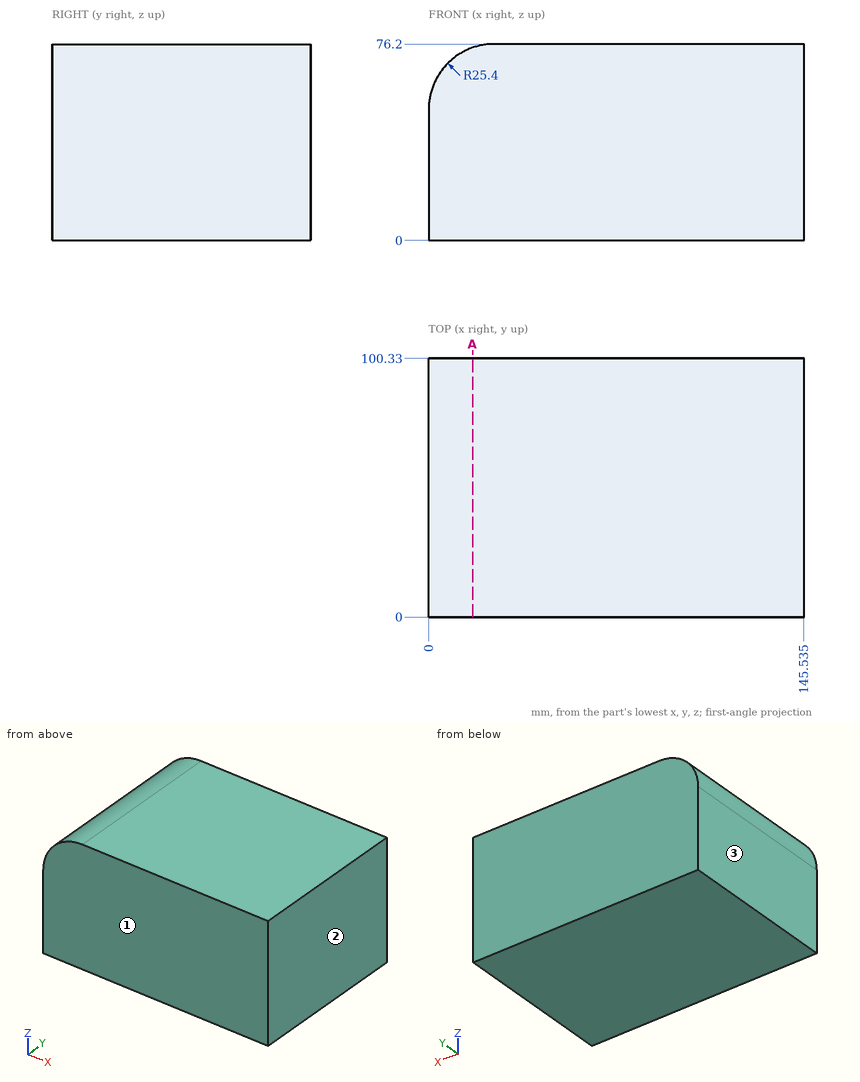
Part print with two shaded views. Sizes in mm from the minimum x, y, z corner. Round coordinates to 2 decimals unless told otherwise and drop trailing zeros. Write each loop counter-clockwise with the first axis right and the second up, starting at its lowest first coordinate (ties: lowest second). Pieces come first, ordered by that corner, then holes. Notation, with made-up numbers: (76.5, 43) - (84.5, 43) arc R18 cw to (84.5, 69) - close; hole circle Ø6 at (42.25, -19). An arc over 180 degrees is marked (long way). Use CSV: the item, a comma, the result in double quotes.
Item 1: Flat gauge pins, fed straight in: P1, Ø2, axis at x = 130, y = 79, coming from the -Z side; P2, Ø1, axis at y = 24, z = 67, coming from the -X side. Where does each tip first touch, or does it go through?
Results list:
P1,"stops at z = 0"
P2,"stops at x = 5.43"
Item 2: Pull direction X, two halves, no side cores. Call the marked faces 1, 2 and 3: pulls with the +X half, pulls with the -X half, needs draft (parallel to the pull), parting line crosses it, or undercut.
Results list:
face 1,"needs draft"
face 2,"pulls with the +X half"
face 3,"pulls with the -X half"
Item 3: Slice it at A-A, the plane x = 17. Write the cut outline in (y, z).
Results list:
outline,"(0, 0) - (100.33, 0) - (100.33, 74.77) - (0, 74.77) - close"
Item 4: Wall check: L1, parallel to X at y = 8, z = 53.5 (3 decimals); L2, parallel to X at y = 81.5, z = 60.5 (1 decimal). Give the ranges that are in metal, low to high.
Results list:
L1,"x = 0.144 to 145.535"
L2,"x = 1.9 to 145.5"
